Check sheet for the modelled part. Datum: model origin and axes. Units: mm. Give positions to 0.01 mm unless a question says otherwise; leave off trailing zeros. Write each loop counter-clockwise with the first axis right and the second up, starting at its lowest first coordinate (ties: lowest second). Pieces come first, ordered by that corner, then holes. Notation, with made-up numbers: (10, 69) -> (19, 69) arc R22 ccw to (19, 107) -> close; hole circle Ø8 at (-1.5, -39.75). An arc over 180 degrees is marked (long way). Answer as a JSON object with one key per item and string values.
Autodesk Inventor part; units mm, degrees
ref_plane "YZ Plane" through (0, 0, 0) normal (1, 0, 0) x (0, 1, 0)
ref_plane "XZ Plane" through (0, 0, 0) normal (0, 1, 0) x (-1, 0, 0)
ref_plane "XY Plane" through (0, 0, 0) normal (0, 0, 1) x (1, 0, 0)
sketch "Sketch1" plane through (0, 0, 0) normal (0, 0, 1) x (1, 0, 0)
  line L0 (-6.35, 0) -> (6.35, 0)
  line L1 (-6.35, -2.3876) -> (6.35, -2.3876)
  line L2 (6.35, 0) -> (6.35, 17.8562)
  line L3 (6.35, 17.8562) -> (8.7376, 17.8562)
  line L4 (8.7376, 17.8562) -> (8.7376, -20.2438)
  line L5 (8.7376, -20.2438) -> (6.35, -20.2438)
  line L6 (6.35, -20.2438) -> (6.35, -2.3876)
  line L7 (-6.35, -2.3876) -> (-6.35, -20.2438)
  line L8 (-6.35, -20.2438) -> (-8.7376, -20.2438)
  line L9 (-8.7376, -20.2438) -> (-8.7376, 17.8562)
  line L10 (-8.7376, 17.8562) -> (-6.35, 17.8562)
  line L11 (-6.35, 17.8562) -> (-6.35, 0)
  point P0 (0, 0)
  point P1 (0, 0)
  dimension "d9" = 12.7
  dimension "d10" = 2.3876
  dimension "d11" = 17.8562
  dimension "d12" = 38.1
  dimension "d13" = 2.3876
  dimension "d14" = 2.3876
  dimension "d15" = 2.3876
  dimension "d16" = 17.8562
  dimension "d17" = 17.8562
extrude "Extrusion1" add sketch "Sketch1" against normal blind 203.2
sketch "Sketch2" plane through (8.7376, -20.2438, 0) normal (1, 0, 0) x (0, 0, -1)
  point P0 (0, 0)
  point P1 (9.525, 6.35)
  dimension "d20" = 9.525
  dimension "d21" = 6.35
hole "Hole1" at (8.7376, -13.8938, -9.525) direction (-1, 0, 0) diameter 4.2164 end through all
sketch "Sketch3" plane through (8.7376, -20.2438, 0) normal (1, 0, 0) x (0, 0, -1)
  point P0 (0, 38.1)
  point P1 (9.525, 23.0188)
  dimension "d29" = 15.0813
  dimension "d30" = 9.525
hole "Hole2" at (8.7376, 2.775, -9.525) direction (-1, 0, 0) diameter 4.2164 end through all
sketch "Sketch4" plane through (8.7376, -20.2438, 0) normal (1, 0, 0) x (0, 0, -1)
  circle A0 centre (9.525, 23.0188) radius 2.1082
  circle A1 centre (9.525, 6.35) radius 2.1082
  line L0 (0, 0) -> (203.2, 0)
  line L1 (0, 38.1) -> (203.2, 38.1)
  line L2 (101.6, 38.1) -> (101.6, 0) construction
  circle A2 centre (193.675, 23.0188) radius 2.1082
  circle A3 centre (193.675, 6.35) radius 2.1082
hole "Hole3" at (8.7376, 2.775, -193.675) at (8.7376, -13.8938, -193.675) direction (-1, 0, 0) diameter 4.2164 end through all
sketch "Sketch5" plane through (8.7376, -20.2438, 0) normal (1, 0, 0) x (0, 0, -1)
  line L0 (19.05, 5.08) -> (38.1, 5.08)
  line L1 (41.275, 8.255) -> (41.275, 14.605)
  line L2 (38.1, 17.78) -> (19.05, 17.78)
  line L3 (15.875, 14.605) -> (15.875, 8.255)
  arc A0 (19.05, 17.78) -> (15.875, 14.605) centre (19.05, 14.605) ccw
  arc A1 (41.275, 14.605) -> (38.1, 17.78) centre (38.1, 14.605) ccw
  arc A2 (38.1, 5.08) -> (41.275, 8.255) centre (38.1, 8.255) ccw
  arc A3 (15.875, 8.255) -> (19.05, 5.08) centre (19.05, 8.255) ccw
  point P0 (0, 0)
  point P1 (41.275, 17.78)
  point P2 (41.275, 5.08)
  point P3 (15.875, 17.78)
  point P4 (28.575, 17.78)
  point P5 (28.575, 17.78)
  dimension "d45" = 25.4
  dimension "d46" = 12.7
  dimension "d47" = 17.78
  dimension "d48" = 28.575
  dimension "d49" = 3.175
extrude "Extrusion2" cut sketch "Sketch5" against normal through all
sketch "Sketch6" plane through (8.7376, -20.2438, 0) normal (1, 0, 0) x (0, 0, -1)
  arc A0 (19.05, 17.78) -> (15.875, 14.605) centre (19.05, 14.605) ccw
  arc A1 (41.275, 14.605) -> (38.1, 17.78) centre (38.1, 14.605) ccw
  arc A2 (38.1, 5.08) -> (41.275, 8.255) centre (38.1, 8.255) ccw
  arc A3 (15.875, 8.255) -> (19.05, 5.08) centre (19.05, 8.255) ccw
  line L0 (101.6, 38.1) -> (101.6, 0) construction
  arc A4 (187.325, 14.605) -> (184.15, 17.78) centre (184.15, 14.605) ccw
  line L1 (184.15, 17.78) -> (165.1, 17.78)
  arc A5 (165.1, 17.78) -> (161.925, 14.605) centre (165.1, 14.605) ccw
  line L2 (161.925, 14.605) -> (161.925, 8.255)
  arc A6 (161.925, 8.255) -> (165.1, 5.08) centre (165.1, 8.255) ccw
  line L3 (165.1, 5.08) -> (184.15, 5.08)
  arc A7 (184.15, 5.08) -> (187.325, 8.255) centre (184.15, 8.255) ccw
  line L4 (187.325, 8.255) -> (187.325, 14.605)
extrude "Extrusion3" cut sketch "Sketch6" against normal through all
sketch "Sketch7" plane through (-6.35, 0, 0) normal (0, 1, 0) x (1, 0, 0)
  line L0 (15.0876, 19.05) -> (15.0876, 38.1)
  line L1 (-2.3876, 38.1) -> (-2.3876, 19.05)
  line L2 (-2.3876, 28.575) -> (15.0876, 28.575) construction
  line L3 (-2.3876, 28.575) -> (6.35, 28.575) construction
  dimension "d54" = 17.4752
hole "Hole4" at (0, 0, -28.575) direction (0, -1, 0) diameter 4.2164 end through all
sketch "Sketch8" plane through (-6.35, 0, 0) normal (0, 1, 0) x (1, 0, 0)
  circle A0 centre (6.35, 28.575) radius 2.1082
  line L0 (0, 0) -> (0, 203.2)
  line L1 (15.0876, 101.6) -> (-2.2502, 101.6)
  circle A1 centre (6.35, 174.625) radius 2.1082
hole "Hole5" at (0, 0, -174.625) direction (0, -1, 0) diameter 4.2164 end through all
sketch "Sketch9" plane through (8.7376, -20.2438, 0) normal (1, 0, 0) x (0, 0, -1)
  line L0 (0, 20.2438) -> (203.2, 20.2438)
  line L1 (101.6, 38.1) -> (101.6, 0) construction
  line L2 (50.8, 20.2438) -> (152.4, 20.2438)
  line L3 (155.575, 23.4188) -> (155.575, 23.4188)
  line L4 (152.4, 26.5938) -> (50.8, 26.5938)
  line L5 (47.625, 23.4188) -> (47.625, 23.4188)
  arc A0 (50.8, 26.5938) -> (47.625, 23.4188) centre (50.8, 23.4188) ccw
  arc A1 (47.625, 23.4188) -> (50.8, 20.2438) centre (50.8, 23.4188) ccw
  arc A2 (155.575, 23.4188) -> (152.4, 26.5938) centre (152.4, 23.4188) ccw
  arc A3 (152.4, 20.2438) -> (155.575, 23.4188) centre (152.4, 23.4188) ccw
  point P0 (155.575, 26.5938)
  point P1 (155.575, 20.2438)
  point P2 (47.625, 26.5938)
  point P3 (101.6, 20.2438)
  dimension "d69" = 107.95
  dimension "d70" = 6.35
  dimension "d71" = 3.175
extrude "Extrusion4" cut sketch "Sketch9" against normal through all
equation "\"d13\" = d10"
equation "\"d14\" = d10"
equation "\"d15\" = d10"
equation "\"d16\" = d11"
equation "\"d17\" = d11"
properties part number "car frame"
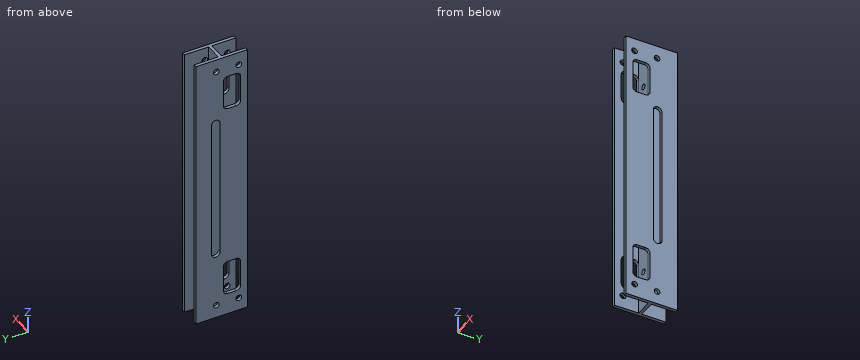
1. Sectioned sample at B-B, the plane y = 10.5. Enter the section's corners in (x, z).
Determined:
{"outline": "(-8.74, -203.2) -> (-6.35, -203.2) -> (-6.35, 0) -> (-8.74, 0) -> close; (6.35, -203.2) -> (8.74, -203.2) -> (8.74, 0) -> (6.35, 0) -> close"}
2. Go/stop test with flat-tipped pins: P1, Ø1.5, axis at x = 4, y = 6.5, coming from the +Z side; P2, Ø8, axis at x = 1.5, z = -54, coming from the +Y side. Record where each tip stops, or that it passes through.
Determined:
{"P1": "through", "P2": "y = 0"}
3. Scan lines: L1, parallel to Z at x = 0, y = -1.4; L2, parallel to Y at x = -7.5, z = -62.5; L3, parallel to X at y = 11.5, z = -113.5. Record each from-to range of solid material in increasing order. Write a range as [from, to].
Determined:
{"L1": "[-203.2, -176.73], [-172.52, -30.68], [-26.47, 0]", "L2": "[-20.24, 0], [6.35, 17.86]", "L3": "[-8.74, -6.35], [6.35, 8.74]"}
4. Sectioned sample at A-A, the plane x = 0. Enter the section's corners in (y, z), plus the area to 3 significant figures.
Determined:
{"outline": "(-2.39, -203.2) -> (0, -203.2) -> (0, -176.73) -> (-2.39, -176.73) -> close; (-2.39, -172.52) -> (0, -172.52) -> (0, -30.68) -> (-2.39, -30.68) -> close; (-2.39, -26.47) -> (0, -26.47) -> (0, 0) -> (-2.39, 0) -> close", "area": "465 mm^2"}
